Geometry check sheet. Reference: drawing and pictorial views, mm from the part's lowest x, y, z. A direction names the side the tool comes from. Give positions to 0.01 mm unless a question says otherwise; leave off trailing zeros. Order: outer loops, then holes, each group sorted by start corner. A loop starts at its lowest first (then second) coordinate and runs counter-clockwise, first axis right, second up.
Item 1: Sectioned sample at A-A on x = 90. Record the boundary of the cut face in (y, z), and give its area (3 significant figures).
Item 2: Gauge pin test, flat ends, axial feed: P1, Ø13, axis at x = 90, z = 10, coming from the -Y side; P2, Ø10, axis at x = 32, y = 4.5, coming from the -Z side; P3, Ø4, axis at x = 64.5, z = 90.5, coming from the -Y side. Record the tip position at first contact, or that the pin passes through.
Item 3: Material ranges on line 1 along Z through (x, y) = (74.5, 15.75); line 2 along Z through (x, y) = (28.5, 2.5); line 3 along Z through (x, y) = (90, 21), recorded low to high.
Item 4: Sectioned sample at C-C on y = 11. Record the boundary of the cut face in (x, z).
Item 5: Sectioned sample at B-B on z = 10. Record the boundary of the cut face in (x, y), and give its area (3 significant figures).
Item 6: Sectioned sample at D-D on x = 19.5. Record the boundary of the cut face in (y, z).
Item 7: Access from +Z, -Z, +X, -X, +Y, -Y to the whole of each face (thin tool, end or side, straight path). Record for the marked faces 1 and 2.
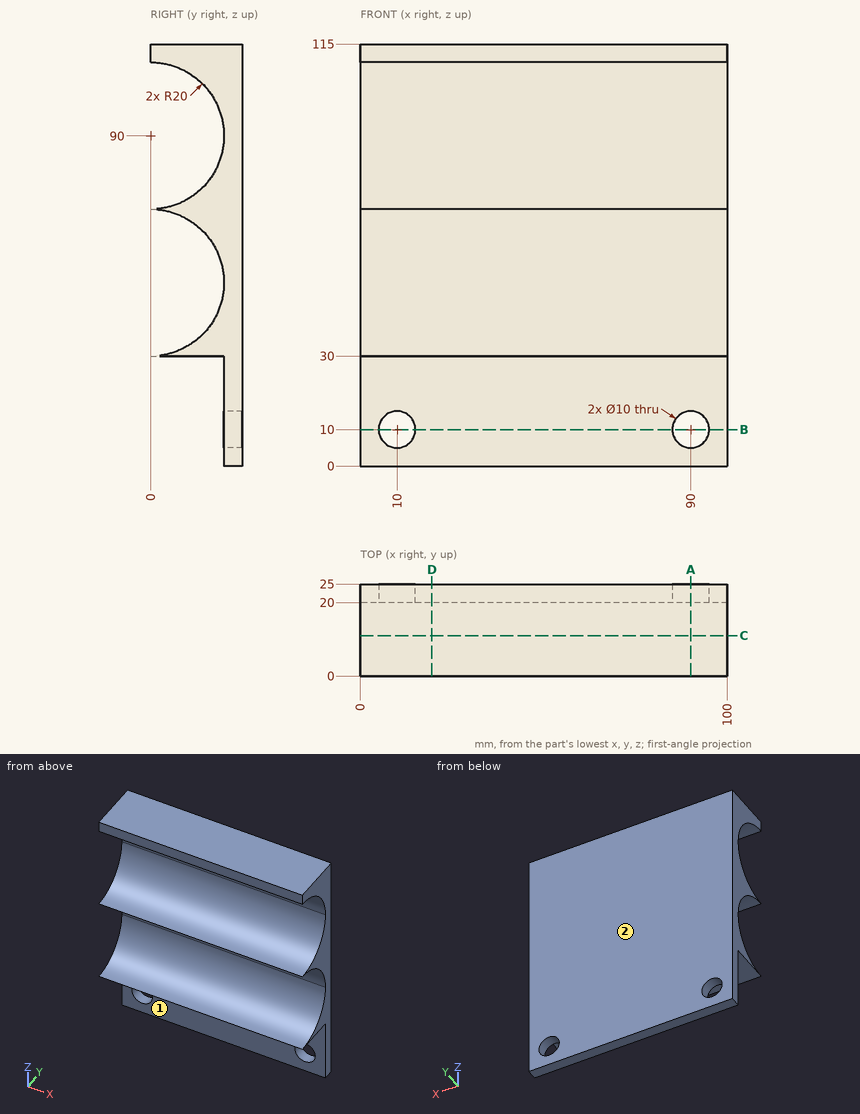
Report:
1. outline: (0, 30) - (20, 30) - (20, 15) - (25, 15) - (25, 115) - (0, 115) - (0, 110) arc R20 cw to (20, 90) arc R20 cw to (0, 70) arc R20 cw to (20, 50) arc R20 cw to start; (20, 0) - (25, 0) - (25, 5) - (20, 5) - close
1. area: 968 mm2
2. P1: stops at y = 20
2. P2: stops at z = 30
2. P3: stops at y = 19.84
3. line 1: z = 30 to 37.67, 62.33 to 77.67, 102.33 to 115
3. line 2: z = 30 to 30.16, 69.84 to 70.16, 109.84 to 115
3. line 3: z = 0 to 5, 15 to 115
4. outline: (0, 30) - (100, 30) - (100, 33.3) - (0, 33.3) - close; (0, 66.7) - (100, 66.7) - (100, 73.3) - (0, 73.3) - close; (0, 106.7) - (100, 106.7) - (100, 115) - (0, 115) - close
5. outline: (0, 20) - (5, 20) - (5, 25) - (0, 25) - close; (15, 20) - (85, 20) - (85, 25) - (15, 25) - close; (95, 20) - (100, 20) - (100, 25) - (95, 25) - close
5. area: 400 mm2
6. outline: (0, 30) - (20, 30) - (20, 0) - (25, 0) - (25, 115) - (0, 115) - (0, 110) arc R20 cw to (20, 90) arc R20 cw to (0, 70) arc R20 cw to (20, 50) arc R20 cw to start
7. face 1: -Z, +X, -X, -Y
7. face 2: +Z, -Z, +X, -X, +Y
